The model under review builds one solid part; all positions refer to its coordinate system, in mm. A direction names the side the tool comes from. Round coordinates to 2 decimals unless told otherwise and drop trailing zeros. Order: outer loops, then holes, each group sorted by start corner. A loop starts at its lowest first (then second) coordinate and runs counter-clockwise, first axis right, second up.
1) Consider section C-C (x = -3.5). Give the boundary of the cut face in (y, z), then the cut area to 3 significant figures.
2) Consider section D-D (z = 30). Give the boundary of the cut face in (x, y), then the cut area to 3 significant figures.
3) To check wall thickness, follow L1, parallel to Z at x = 9.75, y = 12.7; L2, parallel to Z at x = 24.5, y = 19; L3, parallel to X at y = 8, z = 11.5. State the ranges of each line that lie inside material, in increasing order.
4) Consider section A-A (y = 14.75). Give the boundary of the cut face in (x, z), then the cut area to 3 significant figures.
5) Mouldability with a two-part tool opening along Y and no side actions: class faces 1 (the face through (2, 0, 12)), 2 (the face through (21.7, 15.7, 12.7)), 3 (the face through (22.9, 17, 6.4)) as pulls with the +Y half, pulls with the -Y half, needs draft (parallel to the pull), parting line crosses it, or undercut.
6) Clearance check with flat-ended pins moving along their axes: P1, Ø6, axis at x = -25, z = 17, coming from the -Y side; P2, Ø7.5, axis at y = 18.5, z = 21, coming from the -X side; P3, Ø1, axis at x = 11.5, y = 20, coming from the +Z side; P4, Ø12.5, axis at x = -26, y = 18, coming from the +Z side. State where each tip first meets the part, or that it passes through.
7) Machinability: for faces 4 (the face through (-20, 19, 12.7)), 5 (the face through (39.97, 12.98, 6.44)), 6 (the face through (14.874, 13, 24)), which of the approach directions +Z, -Z, +X, -X, +Y, -Y give a long, thin tool a straight path to every point of the face, cutting with its end or side? Answer none if there is none.
from build123d import *

# Parameters (mm, degrees)
F0_W      = 76.2
F0_H      = 25.4
F1_DEPTH  = 12.7
F2_R      = 6.35
F3_DEPTH  = 25.4
F4_W      = 25.4
F4_H      = 25.4
F5_DEPTH  = 31.75
F7_DEPTH  = 25.4
F9_DEPTH  = 25.4
F10_R     = 6.35
F11_DEPTH = 25.4
F13_DEPTH = 25.4


with BuildPart() as f1:
    # F0 (on Top) → F1 (new body)
    with BuildSketch(Plane.XY):
        with Locations((2.1738717566, 12.7)):
            Rectangle(F0_W, F0_H)
    extrude(amount=F1_DEPTH)

    # F2 (on face) → F3 (cut)
    with BuildSketch(Plane.XY.offset(12.7)):
        with Locations((-23.2261282434, 12.7)):
            Circle(F2_R)
        with Locations((27.5738717566, 12.7)):
            Circle(F2_R)
    extrude(amount=-F3_DEPTH, mode=Mode.SUBTRACT)

    # F4 (on face) → F5 (join)
    with BuildSketch(Plane.XY.offset(12.7)):
        with Locations((2.1738717566, 12.7)):
            Rectangle(F4_W, F4_H)
    extrude(amount=F5_DEPTH)

    # F6 (on face) → F7 (cut)
    with BuildSketch(Plane.XY.offset(12.7)):
        with BuildLine():
            ThreePointArc((27.5738717566, 25.4), (39.9715783926, 12.7), (27.5738717566, 0))
            Line((27.5738717566, 0), (40.2738717566, 0))
            Line((40.2738717566, 0), (40.2738717566, 25.4))
            Line((40.2738717566, 25.4), (27.5738717566, 25.4))
        make_face()
    extrude(amount=-F7_DEPTH, mode=Mode.SUBTRACT)

    # F8 (on face) → F9 (cut)
    with BuildSketch(Plane.XY.offset(12.7)):
        with BuildLine():
            ThreePointArc((-23.2261282434, 0), (-35.6730291754, 12.7), (-23.2261282434, 25.4))
            Line((-23.2261282434, 25.4), (-35.9261282434, 25.4))
            Line((-35.9261282434, 25.4), (-35.9261282434, 0))
            Line((-35.9261282434, 0), (-23.2261282434, 0))
        make_face()
    extrude(amount=-F9_DEPTH, mode=Mode.SUBTRACT)

    # F10 (on face) → F11 (cut)
    with BuildSketch(Plane.YZ.offset(14.8738717566)):
        with Locations((12.7, 31.75)):
            Circle(F10_R)
    extrude(amount=-F11_DEPTH, mode=Mode.SUBTRACT)

    # F12 (on face) → F13 (cut)
    with BuildSketch(Plane.YZ.offset(14.8738717566)):
        with BuildLine():
            ThreePointArc((0, 31.75), (12.7, 43.5445759726), (25.4, 31.75))
            Line((25.4, 31.75), (25.4, 44.45))
            Line((25.4, 44.45), (0, 44.45))
            Line((0, 44.45), (0, 31.75))
        make_face()
    extrude(amount=-F13_DEPTH, mode=Mode.SUBTRACT)


solid = f1.part
Answer below:
1. outline: (0, 0) - (25.4, 0) - (25.4, 31.75) arc R12.73 ccw to (0, 31.75) - close; hole circle Ø12.7 at (12.7, 31.75)
1. area: 911 mm2
2. outline: (-10.53, 0) - (14.87, 0) - (14.87, 6.6) - (-10.53, 6.6) - close; (-10.53, 18.8) - (14.87, 18.8) - (14.87, 25.4) - (-10.53, 25.4) - close
2. area: 335 mm2
3. L1: z = 0 to 25.4, 38.1 to 43.54
3. L2: z = 0 to 12.7
3. L3: x = -34.77 to -27.5, -18.96 to 23.3, 31.84 to 39.07
4. outline: (-35.51, 0) - (-29.24, 0) - (-29.24, 12.7) - (-35.51, 12.7) - close; (-17.22, 0) - (21.56, 0) - (21.56, 12.7) - (14.87, 12.7) - (14.87, 25.74) - (-10.53, 25.74) - (-10.53, 12.7) - (-17.22, 12.7) - close; (-10.53, 37.76) - (14.87, 37.76) - (14.87, 43.38) - (-10.53, 43.38) - close; (33.58, 0) - (39.81, 0) - (39.81, 12.7) - (33.58, 12.7) - close
4. area: 1,130 mm2
5. face 1: pulls with the -Y half
5. face 2: needs draft
5. face 3: undercut
6. P1: passes through
6. P2: stops at x = -10.53
6. P3: stops at z = 41.58
6. P4: stops at z = 12.7
7. face 4: +Z, -X, +Y, -Y
7. face 5: +Z, -Z, +X
7. face 6: +Z, +X, +Y, -Y
